Read the model definition and answer for the solid it produces. Units are mm, in the model's axes. Face numbers are marked on the shaded views. Give positions to 0.01 mm unless a question says otherwise; leave off trailing zeros. Write each loop counter-clockwise with the first axis right and the second up, starting at its lowest first coordinate (ties: lowest second). Pieces come first, ordered by that corner, then holes. Notation, with made-up numbers: (72.5, 40.25) -> (101.5, 40.25) arc R15 ccw to (101.5, 69.25) -> close; hole circle Ø8 at (-18, 20). An arc over 180 degrees is marked (long way). Answer as CSV lines item,"result". Start each with the question number.
1. Given pin 1 (2 mm diameter, centred on y = 11, z = 2.5, fed in from +X), flat-ended and moving along its own axis, determine where the tip first touches the part or whether it passes through.
2. Find the intervals of material crossed by line 1 (Y direction, x = 0, z = 5.25); line 2 (Y direction, x = 0, z = 4.5); line 3 (Y direction, x = 0, z = 3.25), in increasing order.
3. The part is cut by section A-A, the plane y = 0. Determine the outline of the cut face in (x, z), and give its area (3 significant figures).
4. The part is cut by section B-B, the plane x = 0. Determine the outline of the cut face in (y, z).
5. For a pull along X with two mould halves and no side action, classify the marked faces 1, 2 and 3 as pulls with the +X half, pulls with the -X half, needs draft (parallel to the pull), parting line crosses it, or undercut.
6. The part is cut by section C-C, the plane z = 1.75. Determine the outline of the cut face in (x, y).
7. The part is cut by section D-D, the plane z = 5.75. Determine the outline of the cut face in (x, y), and give its area (3 significant figures).
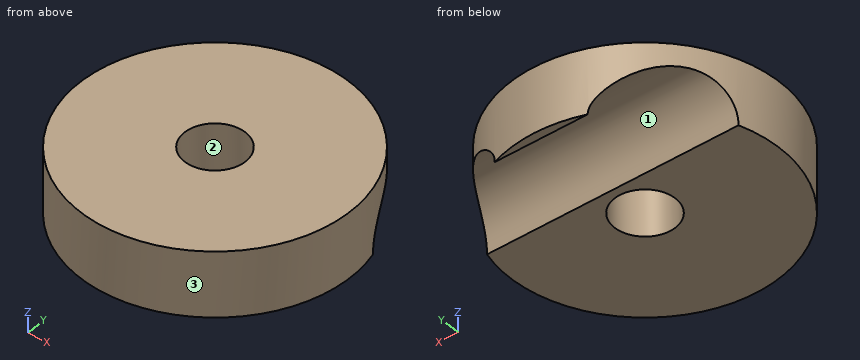
from build123d import *

# Parameters (mm, degrees)
F0_R     = 15.5
F2_DEPTH = 7.5
F3_R     = 5
F4_DEPTH = 20
F5_D     = 7


with BuildPart() as f2:
    # F0 (on Top) → F2 (new body)
    with BuildSketch(Plane.XY):
        Circle(F0_R)
    extrude(amount=F2_DEPTH)

    # F3 (on Right) → F4 (cut, symmetric)
    with BuildSketch(Plane.YZ):
        with Locations((9.5, 0)):
            Circle(F3_R)
    extrude(amount=F4_DEPTH, both=True, mode=Mode.SUBTRACT)

    # F5 (through all)
    with Locations(Plane(origin=(0, 0, 0), x_dir=(1, 0, 0), z_dir=(0, 0, -1))):
        with Locations((0, 0)):
            Hole(F5_D / 2)


solid = f2.part
Results found:
1,pin 1,"passes through"
2,line 1,"y = -15.5 to -3.5, 3.5 to 15.5"
2,line 2,"y = -15.5 to -3.5, 3.5 to 7.32, 11.68 to 15.5"
2,line 3,"y = -15.5 to -3.5, 3.5 to 5.7, 13.3 to 15.5"
3,outline,"(-15.5, 0) -> (-3.5, 0) -> (-3.5, 7.5) -> (-15.5, 7.5) -> close; (3.5, 0) -> (15.5, 0) -> (15.5, 7.5) -> (3.5, 7.5) -> close"
3,area,"180 mm²"
4,outline,"(-15.5, 0) -> (-3.5, 0) -> (-3.5, 7.5) -> (-15.5, 7.5) -> close; (3.5, 0) -> (4.5, 0) arc R5 cw to (14.5, 0) -> (15.5, 0) -> (15.5, 7.5) -> (3.5, 7.5) -> close"
5,face 1,"needs draft"
5,face 2,"undercut"
5,face 3,"parting line crosses it"
6,outline,"(-14.73, 4.82) arc R15.5 ccw (long way) to (14.73, 4.82) -> close; (-6.25, 14.18) -> (6.25, 14.18) arc R15.5 ccw to start; hole circle Ø7 at (0, 0)"
7,outline,"circle Ø31 at (0, 0); hole circle Ø7 at (0, 0)"
7,area,"716 mm²"
